Design review of the part built by this model. Coordinates are the model's own, in mm. Round coordinates to 2 decimals unless told otherwise and drop trailing zeros. Write each loop counter-clockwise with the first axis right and the second up, starting at its lowest first coordinate (ties: lowest second). Pieces come first, ordered by that corner, then holes.
from build123d import *

# Parameters (mm, degrees)
F0_R     = 5.625
F0_R_2   = 2.675
F1_DEPTH = 14
F2_DEPTH = 4


with BuildPart() as f1:
    # F0 (on Top) → F1 (new body)
    with BuildSketch(Plane.XY):
        with Locations((-25, 0)):
            Circle(F0_R)
        with Locations((-25, 0)):
            Circle(F0_R_2, mode=Mode.SUBTRACT)
        with Locations((25, 0)):
            Circle(F0_R)
        with Locations((25, 0)):
            Circle(F0_R_2, mode=Mode.SUBTRACT)
    extrude(amount=F1_DEPTH)

    # F0 (on Top) → F2 (join)
    with BuildSketch(Plane.XY):
        with BuildLine():
            Line((31.625, 8.075), (-31.625, 8.075))
            ThreePointArc((-31.625, 8.075), (-35.160534, 6.610534), (-36.625, 3.075))
            Line((-36.625, 3.075), (-36.625, -0.925))
            ThreePointArc((-36.625, -0.925), (-35.160534, -4.460534), (-31.625, -5.925))
            Line((-31.625, -5.925), (31.625, -5.925))
            ThreePointArc((31.625, -5.925), (35.160534, -4.460534), (36.625, -0.925))
            Line((36.625, -0.925), (36.625, 3.075))
            ThreePointArc((36.625, 3.075), (35.160534, 6.610534), (31.625, 8.075))
        make_face()
        with Locations((-25, 0)):
            Circle(F0_R, mode=Mode.SUBTRACT)
        with Locations((25, 0)):
            Circle(F0_R, mode=Mode.SUBTRACT)
        with Locations((-25, 0)):
            Circle(F0_R)
        with Locations((-25, 0)):
            Circle(F0_R_2, mode=Mode.SUBTRACT)
        with Locations((25, 0)):
            Circle(F0_R)
        with Locations((25, 0)):
            Circle(F0_R_2, mode=Mode.SUBTRACT)
    extrude(amount=-F2_DEPTH)


solid = f1.part
1) Add section C-C on z = 6.25. State the section outline as (x, y) points (3 decimals).
2) Add section D-D on y = -5. State the section outline as (x, z) points, and give its area (3 significant figures).
3) Add section A-A on x = 25. State the section outline as (y, z) points (3 decimals).
4) For line 1 along X through (y, z) = (1, 12.75); line 2 along X through (y, z) = (1.5, 10); line 3 along Y through (x, z) = (-25, 10.5) (3 decimals), list the stretches that pass through material, from the lowest coordinate up.
5) Add section B-B on y = 0. State the section outline as (x, z) points (3 decimals).
6) The part is to be moulded in two halves that separate along X. For faces 1 (the face through (19.38, 0.25, 6.9)), 2 (the face through (35.12, -4.5, -1.97)), 3 (the face through (0, -5.925, -2)), 4 (the face through (-30.62, 0.25, 6.9)), say which applies: pulls with the +X half, pulls with the -X half, needs draft (parallel to the pull), parting line crosses it, or undercut.
7) For P1, Ø5, axis at y = 6.5, z = 6, coming from the -X side; P2, Ø1.5, axis at y = 4, z = 5, coming from the +X side, all flat-tipped, find the tip position at first contact; note any pin that passes through.
Computed:
1. outline: circle Ø11.25 at (-25, 0); circle Ø11.25 at (25, 0); hole circle Ø5.35 at (-25, 0); hole circle Ø5.35 at (25, 0)
2. outline: (-34.52, -4) - (34.52, -4) - (34.52, 0) - (27.58, 0) - (27.58, 14) - (22.42, 14) - (22.42, 0) - (-22.42, 0) - (-22.42, 14) - (-27.58, 14) - (-27.58, 0) - (-34.52, 0) - close
2. area: 420 mm2
3. outline: (-5.925, -4) - (-2.675, -4) - (-2.675, 14) - (-5.625, 14) - (-5.625, 0) - (-5.925, 0) - close; (2.675, -4) - (8.075, -4) - (8.075, 0) - (5.625, 0) - (5.625, 14) - (2.675, 14) - close
4. line 1: x = -30.54 to -27.48, -22.52 to -19.46, 19.46 to 22.52, 27.48 to 30.54
4. line 2: x = -30.42 to -27.21, -22.79 to -19.58, 19.58 to 22.79, 27.21 to 30.42
4. line 3: y = -5.625 to -2.675, 2.675 to 5.625
5. outline: (-36.625, -4) - (-27.675, -4) - (-27.675, 14) - (-30.625, 14) - (-30.625, 0) - (-36.625, 0) - close; (-22.325, -4) - (22.325, -4) - (22.325, 14) - (19.375, 14) - (19.375, 0) - (-19.375, 0) - (-19.375, 14) - (-22.325, 14) - close; (27.675, -4) - (36.625, -4) - (36.625, 0) - (30.625, 0) - (30.625, 14) - (27.675, 14) - close
6. face 1: undercut
6. face 2: pulls with the +X half
6. face 3: needs draft
6. face 4: undercut
7. P1: stops at x = -28.95
7. P2: stops at x = 29.59
